from build123d import *

# Parameters (mm, degrees)
SKETCH1_R           = 2.25
BOSS_EXTRUDE1_DEPTH = 10
BOSS_EXTRUDE1_TAPER = 5
SKETCH1_3_R         = 1.375
BOSS_EXTRUDE2_DEPTH = 1
SKETCH5_R           = 1.25
BOSS_EXTRUDE3_DEPTH = 1
SKETCH6_R           = 2.25
BOSS_EXTRUDE4_DEPTH = 2
SKETCH14_R          = 1.274517671
BOSS_EXTRUDE6_DEPTH = 33
SKETCH15_R          = 1.274517671
BOSS_EXTRUDE8_DEPTH = 2
BOSS_EXTRUDE8_TAPER = -26
SKETCH17_R          = 2.25
BOSS_EXTRUDE9_DEPTH = 17
SKETCH18_R          = 1.4
CUT_EXTRUDE2_DEPTH  = 15


with BuildPart() as part:
    # Sketch1 → Boss-Extrude1 (new body)
    with BuildSketch(Plane(origin=(0, 0, 0), x_dir=(1, 0, 0), z_dir=(0, 1, 0))):
        with Locations((-0.522013312, 0.511138034)):
            Circle(SKETCH1_R)
    extrude(amount=BOSS_EXTRUDE1_DEPTH, taper=BOSS_EXTRUDE1_TAPER)

    # Sketch1_3 → Boss-Extrude2 (add)
    with BuildSketch(Plane(origin=(0, 0, 0), x_dir=(1, 0, 0), z_dir=(0, 1, 0))):
        with Locations((-0.522013312, 0.511138034)):
            Circle(SKETCH1_3_R)
    extrude(amount=BOSS_EXTRUDE2_DEPTH)

    # Sketch5 → Boss-Extrude3 (add)
    with BuildSketch(Plane.XZ):
        with Locations((-0.522013312, -0.511138034)):
            Circle(SKETCH5_R)
    extrude(amount=BOSS_EXTRUDE3_DEPTH)

    # Sketch6 → Boss-Extrude4 (add)
    with BuildSketch(Plane.XZ.offset(1)):
        with Locations((-0.522013312, -0.511138034)):
            Circle(SKETCH6_R)
    extrude(amount=BOSS_EXTRUDE4_DEPTH)

    # Sketch14 → Boss-Extrude6 (add)
    with BuildSketch(Plane(origin=(0, 10, 0), x_dir=(1, 0, 0), z_dir=(0, 1, 0))):
        with Locations((-0.522013312, 0.511138034)):
            Circle(SKETCH14_R)
    extrude(amount=BOSS_EXTRUDE6_DEPTH)

    # Sketch15 → Boss-Extrude8 (add)
    with BuildSketch(Plane(origin=(0, 43, 0), x_dir=(1, 0, 0), z_dir=(0, 1, 0))):
        with Locations((-0.522013312, 0.511138034)):
            Circle(SKETCH15_R)
    extrude(amount=BOSS_EXTRUDE8_DEPTH, taper=BOSS_EXTRUDE8_TAPER)

    # Sketch17 → Boss-Extrude9 (add)
    with BuildSketch(Plane(origin=(0, 45, 0), x_dir=(1, 0, 0), z_dir=(0, 1, 0))):
        with Locations((-0.522013312, 0.511138034)):
            Circle(SKETCH17_R)
    extrude(amount=BOSS_EXTRUDE9_DEPTH)

    # Sketch18 → Cut-Extrude2 (cut)
    with BuildSketch(Plane(origin=(0, 62, 0), x_dir=(1, 0, 0), z_dir=(0, 1, 0))):
        with Locations((-0.522013312, 0.511138034)):
            Circle(SKETCH18_R)
    extrude(amount=-CUT_EXTRUDE2_DEPTH, mode=Mode.SUBTRACT)


solid = part.part
Work out the finished part from the listing and answer in its coordinate system (mm). A direction names the side the tool comes from. Coordinates: 2 decimals unless noted, no trailing zeros. Write each loop counter-clockwise with the first axis right and the second up, starting at its lowest first coordinate (ties: lowest second). Pieces come first, ordered by that corner, then holes. Notation, with made-up numbers: M 59.25,-7 L 96.25,-7 A15 ccw 96.25,11 Z; hole C 33.5,-33 d8. An arc over 180 degrees is marked long. Use one line per item in the form item = value. Start each with the question number.
1. Each of these flat-tipped pins is pushed along its axis until it touches: P1, Ø0.8, axis at x = -0.5, z = -1, coming from the +Y side; P2, Ø2, axis at x = -0.5, z = 0, coming from the +Y side; P3, Ø1, axis at x = 0, y = 37.5, coming from the +Z side; P4, Ø2, axis at x = -2, y = 11, coming from the +Z side. Where does it stop, or does it pass through?
2. Straight lines are drawn through the part: probe 1 along Z at (x, y) = (-0.3, 13); probe 2 along Z at (x, y) = (0.2, 56.5); probe 3 along Y at (x, z) = (-1.1, -0.75). For each, find the intervals that lie inside material, in ascending order. Write a range as from..to.
3. A tool of negligible diameter and unlimited length cuts with its end or side. For faces 1 (the face through (-1.514, -0.493, -1.272)), 2 (the face through (-1.633, 54.605, 0.341)), 3 (the face through (-1, -3, 0)), from which of +Z, -Z, +X, -X, +Y, -Y can it reach the whole face along a straight path? Write none if from no direction.
4. The part is cut by section A-A (y = 28.5). Give the vertices of the cut face in (x, z), plus the area to 3 significant figures.
5. The part is cut by section B-B (y = 56.5). Give the vertices of the cut face in (x, z).
6. The part is cut by section C-C (y = 2). Give the vertices of the cut face in (x, z).
7. The mould has two halves that part along Z. Classify faces 4 (the face through (-1, 47, -1)), 5 (the face through (-1.533, 26.269, 0.264)), 6 (the face through (-1, -1, -2)): released by +Z, released by -Z, zero draft, split by the parting line, or undercut.
Evaluation:
q1.P1 = 47
q1.P2 = 62
q1.P3 = 0.76
q1.P4 = 0.67
q2.probe_1 = -1.77..0.74
q2.probe_2 = -2.64..-1.71, 0.69..1.62
q2.probe_3 = -3..47
q3.face_1 = none
q3.face_2 = +Y
q3.face_3 = +Z, -Z, +X, -X, -Y
q4.outline = C -0.52,-0.51 d2.55
q4.area = 5.10 mm^2
q5.outline = C -0.52,-0.51 d4.5; hole C -0.52,-0.51 d2.8
q6.outline = C -0.52,-0.51 d4.15
q7.face_4 = undercut
q7.face_5 = split by the parting line
q7.face_6 = zero draft
